from build123d import *

# Parameters (mm, degrees)
SKETCH_1_W         = 55.25
SKETCH_1_H         = 45
EXTRUDE_1_DEPTH    = 6
HOLE_WIZARD_M3_1_D = 2.5
HOLE_WIZARD_M3_2_D = 2.5


with BuildPart() as part:
    # 草图1 → 凸台-拉伸1 (new body)
    with BuildSketch(Plane.XY):
        Rectangle(SKETCH_1_W, SKETCH_1_H)
    extrude(amount=EXTRUDE_1_DEPTH)

    # M3 螺纹孔1 (through all)
    with Locations(Plane(origin=(0, 22.5, 0), x_dir=(1, 0, 0), z_dir=(0, 1, 0))):
        with Locations((-20, -3), (0, -3), (20, -3)):
            Hole(HOLE_WIZARD_M3_1_D / 2)

    # M3 螺纹孔2 (through all)
    with Locations(Plane.ZY.offset(27.625)):
        with Locations((3, 12), (3, -12), (3, 0)):
            Hole(HOLE_WIZARD_M3_2_D / 2)


solid = part.part
Geometry check sheet. Reference: the model listing, model coordinates, mm. Give positions to 0.01 mm unless a question says otherwise; leave off trailing zeros. Write each loop counter-clockwise with the first axis right and the second up, starting at its lowest first coordinate (ties: lowest second). Pieces come first, ordered by that corner, then holes. Notation, with made-up numbers: M 77.5,-31 L 126.5,-31 A16 ccw 126.5,-3 Z; hole C 58,21 d7. An arc over 180 degrees is marked long. Answer as CSV lines item,"result". Start each with the question number.
Q1. Section check C-C, the plane z = 3. Give the number of separate pieces and of enclosed holes in the cut face, then the cut area to 3 significant figures.
Q2. Release check for a two-part mould opening along Z. For faces 1 (the face through (-27.625, -0.3, 1.6)), 2 (the face through (0, 0, 0)), 3 (the face through (-20.577, -17.323, 4.109)) record: pulls with the +Z half, pulls with the -Z half, needs draft (parallel to the pull), parting line crosses it, or undercut.
Q3. Material ranges on L1, parallel to Y at x = 22, z = 3; L2, parallel to Z at x = 20, y = 20; L3, parallel to Y at x = 6.5, z = 2.1, recorded low to high.
Q4. Section check B-B, the plane x = 22. Record the cut outline in (y, z), then the cut area to 3 significant figures.
Q5. Section check A-A, the plane y = 15. Record the cut outline in (x, z) (3 decimals), then the cut area to 3 significant figures.
Geometry says:
1,separate pieces,"16"
1,enclosed holes,"0"
1,area,"1,790 mm^2"
2,face 1,"needs draft"
2,face 2,"pulls with the -Z half"
2,face 3,"undercut"
3,L1,"-22.5 to -13.25, -10.75 to -1.25, 1.25 to 10.75, 13.25 to 22.5"
3,L2,"0 to 1.75, 4.25 to 6"
3,L3,"-22.5 to -12.87, -11.13 to -0.87, 0.87 to 11.13, 12.87 to 22.5"
4,outline,"M -22.5,0 L 22.5,0 L 22.5,6 L -22.5,6 Z; hole C -12,3 d2.5; hole C 0,3 d2.5; hole C 12,3 d2.5"
4,area,"255 mm^2"
5,outline,"M -27.625,0 L 27.625,0 L 27.625,6 L -27.625,6 Z; hole C -20,3 d2.5; hole C 0,3 d2.5; hole C 20,3 d2.5"
5,area,"317 mm^2"
